Input: part model. Units: mm. Frame: model coordinates. Face numbers are marked on the shaded views. A direction names the side the tool comes from. Coordinates: 2 decimals unless noted, no trailing zeros. Write each loop counter-clockwise with the first axis right and the second up, starting at its lowest first coordinate (ties: lowest second). Pieces come first, ordered by that corner, then holes. Notation, with made-up numbers: M 65.5,24 L 115.5,24 A25 ccw 115.5,49 Z; hole C 21.25,-5 d3. An arc over 180 degrees is marked long. Use one line per item in the form item = value.
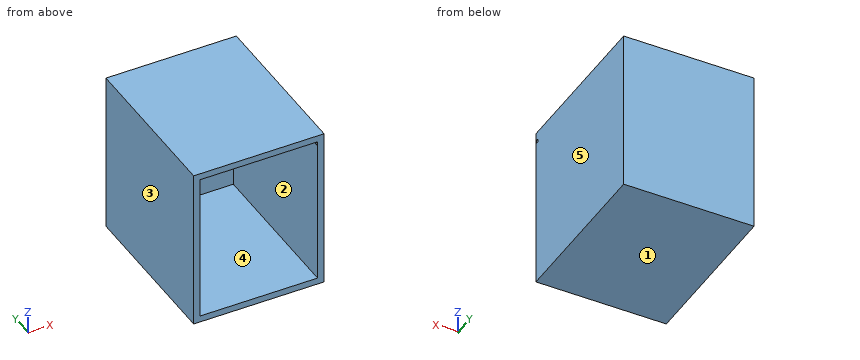
from build123d import *

# Parameters (mm, degrees)
F0_W     = 40
F0_H     = 50
F1_DEPTH = 50
F2_T     = -2
F3_R     = 0.5
F4_DEPTH = 25


with BuildPart() as f1:
    # F0 (on Top) → F1 (new body)
    with BuildSketch(Plane.XY):
        Rectangle(F0_W, F0_H)
    extrude(amount=F1_DEPTH)

    # F2
    f2_openings = [f1.faces().sort_by_distance(p)[0] for p in [
        (0, -25, 25),
    ]]
    offset(amount=F2_T, openings=f2_openings)

    # F3 (on face) → F4 (cut)
    with BuildSketch(Plane(origin=(18, 0, 0), x_dir=(0, -1, 0), z_dir=(-1, 0, 0))):
        with Locations((24.175966, 47.000628)):
            Circle(F3_R)
    extrude(amount=-F4_DEPTH, mode=Mode.SUBTRACT)


solid = f1.part
(1) Set-up query: the marked faces 4 and 5. Return all of +Z, -Z, +X, -X, +Y, -Y with unobstructed straight access to the full face (end or side cutting, diameter ignored); none if empty.
Computed:
face_4 = -Y
face_5 = +Z, -Z, +X, +Y, -Y
(2) Pull-direction query (X, two-part tool) for the marked faces 1, 2 and 3; classes: pulls with the +X half, pulls with the -X half, needs draft (parallel to the pull), parting line crosses it, or undercut.
Computed:
face_1 = needs draft
face_2 = undercut
face_3 = pulls with the -X half
(3) First-contact query: pin 1 Ø4 at (x, z) = (-11, 11.5) entering from -Y. Flat tip, straight axial feed; report the tip coordinate or a pass-through.
Computed:
pin_1 = 23
(4) Section query B-B on x = -12. Return the cut outline in (y, z), plus the area to 3 significant figures.
Computed:
outline = M -25,0 L 25,0 L 25,50 L -25,50 L -25,48 L 23,48 L 23,2 L -25,2 Z
area = 292 mm^2
(5) Section query A-A on y = -12. Return the cut outline in (x, z), plus the area to 3 significant figures.
Computed:
outline = M -20,0 L 20,0 L 20,50 L -20,50 Z; hole M -18,2 L 18,2 L 18,48 L -18,48 Z
area = 344 mm^2
(6) Line query: probe 1 along Z at (x, y) = (14.5, 19.5); probe 2 along X at (y, z) = (-14, 38); probe 3 along Y at (x, z) = (-16.5, 40). Output: solid intervals per line, ascending.
Computed:
probe_1 = 0 to 2, 48 to 50
probe_2 = -20 to -18, 18 to 20
probe_3 = 23 to 25
(7) Section query C-C on z = 7. Return the cut outline in (x, y), plus the area to 3 significant figures.
Computed:
outline = M -20,-25 L -18,-25 L -18,23 L 18,23 L 18,-25 L 20,-25 L 20,25 L -20,25 Z
area = 272 mm^2
